Build history of the part. All positions in model axes, mm. A direction names the side the tool comes from. Give positions to 0.01 mm unless a question says otherwise; leave off trailing zeros. Order: outer loops, then holes, each group sorted by start corner. A loop starts at its lowest first (then second) coordinate and runs counter-clockwise, first axis right, second up. Notation, with made-up numbers: (-38.75, -11) -> (-22.75, -11) arc R23 ccw to (-22.75, 13) -> close; hole circle Ø3 at (-21, -2.75). An arc over 180 degrees is marked (long way). One line per question, with ' | ' between items. Start each with the question number.
(1) Which spindle directions (+Z, -Z, +X, -X, +Y, -Y) get a long thin tool onto all of the face, cutting with end or side? Do faces 1 (the face through (-2.17, 1.67, -2.26)), 2 (the face through (-5, 0, -6)), 3 (the face through (1.2, 0, 5)). Say none if no direction does.
(2) Cut at B-B (x = 0). Give the cut face in (y, z), then the cut area to 3 significant figures.
(3) Drill centre lines: L1, parallel to Y at x = 0, z = 7.5; L2, parallel to Z at x = 1, y = -1; L3, parallel to X at y = -1.25, z = 8.75. Where is each one in solid material? Low to high. Write a range as from..to.
(4) Cut at A-A (y = 0). Give the cut face in (x, z).
(5) Pull direction X, two halves, no side cores. Call faces 4 (the face through (-0.6, 2.71, -2.53)), 5 (the face through (-2, 0, 5)), 6 (the face through (0, 0, 0)), 7 (the face through (0, 0, -7.754)): +X half, -X half, draft (parallel to the pull), parting line (faces both ways), or undercut.
(6) Pin check, flat tip, straight feed: pin 1 Ø4 at (y, z) = (-4, -1) entering from -X. Stop position of the tip, or through.
from build123d import *

# Parameters (mm, degrees)
ESBO_O1_R                = 5
RESSALTO_EXTRUS_O1_DEPTH = 10
RESSALTO_EXTRUS_O3_START = 3
ESBO_O4_R                = 5
RESSALTO_EXTRUS_O3_DEPTH = 3


with BuildPart() as part:
    # Esboço1 → Ressalto-extrusão1 (new body)
    with BuildSketch(Plane.XY):
        Circle(ESBO_O1_R)
        with BuildLine():
            Line((1.2, 1.6), (1.2, -1.6))
            ThreePointArc((1.2, -1.6), (-2, 0), (1.2, 1.6))
        make_face(mode=Mode.SUBTRACT)
    extrude(amount=RESSALTO_EXTRUS_O1_DEPTH)

    # Esboço3 → Revolução1 (revolve)
    with BuildSketch(Plane(origin=(0, 0, 0), x_dir=(1, 0, 0), z_dir=(0, 1, 0))):
        Polygon((0, 0), (5, 0), (2.622856892, 2.377143108), (5, 4.754286215), (0, 4.754286215), align=None)
    revolve(axis=Axis((0, 0, 0), (0, 0, -1)))

    # Esboço4 → Ressalto-extrusão3 (add)
    with BuildSketch(Plane(origin=(0, 0, -4.754286215), x_dir=(-1, 0, 0), z_dir=(0, 0, -1)).offset(RESSALTO_EXTRUS_O3_START)):
        with Locations(Location((0, 0, 0), (0, 0, 180))):
            Circle(ESBO_O4_R)
    extrude(amount=-RESSALTO_EXTRUS_O3_DEPTH)


solid = part.part
Result set:
1) face 1: none | face 2: +Z, -Z | face 3: +Z
2) outline: (-5, -7.75) -> (5, -7.75) -> (5, -4.75) -> (2.62, -2.38) -> (5, 0) -> (5, 10) -> (2, 10) -> (2, 0) -> (-2, 0) -> (-2, 10) -> (-5, 10) -> (-5, 0) -> (-2.62, -2.38) -> (-5, -4.75) -> close | area: 126 mm2
3) L1: y = -5..-2, 2..5 | L2: z = -7.75..0 | L3: x = -4.84..-1.56, 1.2..4.84
4) outline: (-5, -7.75) -> (5, -7.75) -> (5, -4.75) -> (2.62, -2.38) -> (5, 0) -> (5, 10) -> (1.2, 10) -> (1.2, 0) -> (-2, 0) -> (-2, 10) -> (-5, 10) -> (-5, 0) -> (-2.62, -2.38) -> (-5, -4.75) -> close
5) face 4: parting line | face 5: undercut | face 6: undercut | face 7: draft
6) pin 1: stops at x = -4.46
